Design review of the part built by this model. Coordinates are the model's own, in mm. A direction names the side the tool comes from. Round coordinates to 2 decimals unless told otherwise and drop trailing zeros. Order: outer loops, then holes, each group sorted by start corner. A loop starts at its lowest first (then second) coordinate and runs counter-clockwise, first axis right, second up.
Autodesk Fusion 360 part; units mm, degrees
sketch "Sketch1" plane through (0, 0, 0) normal (0, 0, 1) x (1, 0, 0)
  circle A0 centre (0, 0) radius 22.25
  circle A1 centre (0, 0) radius 17.5
  circle A2 centre (0, 0) radius 11
  line L0 (0, 0) -> (0, 30)
  circle A3 centre (0, 17.5) radius 2.6
  circle A4 centre (-15.1554, -8.75) radius 2.6
  circle A5 centre (15.1554, -8.75) radius 2.6
  circle A6 centre (0, 0) radius 3.9
  dimension "d1" = 44.5
  dimension "d2" = 35
  dimension "d3" = 22
  dimension "d4" = 5.2
  dimension "d5" = 5.2
  dimension "d6" = 5.2
  dimension "d7" = 7.8
extrude "Extrude1" add sketch "Sketch1" against normal blind 2.4 contours A0 | A6 | A2 | A1 A3 A4 A5
extrude "Extrude2" add sketch "Sketch1" along normal blind 5 and the other way blind 14 contours A6 | A2
extrude "Extrude3" add sketch "Sketch1" along normal blind 10 contours A6
1) Clearance check with flat-ended pins moving along their axes: P1, Ø6, axis at y = 8.5, z = -5, coming from the +X side; P2, Ø7, axis at x = 0, y = 17.5, coming from the +Z side; P3, Ø4, axis at x = -14.5, y = -9, coming from the -Z side. State where each tip first meets the part, or that it passes through.
Results:
P1: stops at x = 21.12
P2: stops at z = 0
P3: stops at z = -2.4
2) For faces 1 (the face through (5, 10, 0)), 2 (the face through (-2.38, -10.74, -8.12)), 3 (the face through (-16.399, 15.038, -1.183)), list the 3-axis set-ups (+Z, -Z, +X, -X, +Y, -Y) from which the entire face can be reached by the end or side of a thin tool; tool diameter is ignored.
Results:
face 1: +Z
face 2: -Z
face 3: +Z, -Z
3) To check wall thickness, follow line 1 along X through (y, z) = (-8.75, -0.45); line 2 along Y through (x, z) = (0, -0.7); line 3 along Z through (x, y) = (-14, 7). State the ranges of each line that lie inside material, in increasing order.
Results:
line 1: x = -20.46 to -17.76, -12.56 to 12.56, 17.76 to 20.46
line 2: y = -22.25 to 14.9, 20.1 to 22.25
line 3: z = -2.4 to 0
4) Take a section at B-B on y = -7.5. Give the boundary of the cut face in (x, z), plus the area to 3 significant figures.
Results:
outline: (-20.95, -2.4) - (-17.44, -2.4) - (-17.44, 0) - (-20.95, 0) - close; (-12.88, -2.4) - (-8.05, -2.4) - (-8.05, -14) - (8.05, -14) - (8.05, -2.4) - (12.88, -2.4) - (12.88, 0) - (8.05, 0) - (8.05, 5) - (-8.05, 5) - (-8.05, 0) - (-12.88, 0) - close; (17.44, -2.4) - (20.95, -2.4) - (20.95, 0) - (17.44, 0) - close
area: 346 mm2
5) The part is to be moulded in two halves that separate along X. For faces 4 (the face through (-2.38, 10.74, 2.46)), 5 (the face through (13.09, -10.33, -1.18)), 6 (the face through (5, 10, -2.4)), say which applies: released by +X, released by -X, zero draft, split by the parting line, or undercut.
Results:
face 4: split by the parting line
face 5: undercut
face 6: zero draft
6) Take a section at A-A on x = 0. Give the boundary of the cut face in (y, z).
Results:
outline: (-22.25, -2.4) - (-11, -2.4) - (-11, -14) - (11, -14) - (11, -2.4) - (14.9, -2.4) - (14.9, 0) - (11, 0) - (11, 5) - (3.9, 5) - (3.9, 10) - (-3.9, 10) - (-3.9, 5) - (-11, 5) - (-11, 0) - (-22.25, 0) - close; (20.1, -2.4) - (22.25, -2.4) - (22.25, 0) - (20.1, 0) - close
7) Take a section at C-C on y = 16. Give the boundary of the cut face in (x, z), plus the area to 3 significant figures.
Results:
outline: (-15.46, -2.4) - (-2.12, -2.4) - (-2.12, 0) - (-15.46, 0) - close; (2.12, -2.4) - (15.46, -2.4) - (15.46, 0) - (2.12, 0) - close
area: 64.0 mm2
8) Take a section at D-D on y = 9. Give the boundary of the cut face in (x, z).
Results:
outline: (-20.35, -2.4) - (-6.32, -2.4) - (-6.32, -14) - (6.32, -14) - (6.32, -2.4) - (20.35, -2.4) - (20.35, 0) - (6.32, 0) - (6.32, 5) - (-6.32, 5) - (-6.32, 0) - (-20.35, 0) - close
